from build123d import *

# Parameters (mm, degrees)
SKETCH_2_W          = 43.624420354
SKETCH_2_H          = 30
CUT_EXTRUDE_1_DEPTH = 9


with BuildPart() as part:
    # Эскиз1 → Повернуть1 (revolve)
    with BuildSketch(Plane(origin=(0, 0, 0), x_dir=(0, 0, -1), z_dir=(1, 0, 0))):
        Polygon((2.25, 26.387863371), (0, 26.387863371), (0, -1.191709959), (17.25, -1.191709959), (17.25, 65.340178843), (2.55, 65.340178843), (2.55, 50.340178843), (2.25, 50.340178843), align=None)
    revolve(axis=Axis((0, 93.464109616, 0), (0, -1, 0)))

    # Эскиз2 → Вырез-Вытянуть1 (cut)
    with BuildSketch(Plane.XY):
        with Locations((0, 65.340178843)):
            Rectangle(SKETCH_2_W, SKETCH_2_H)
    extrude(amount=-CUT_EXTRUDE_1_DEPTH, mode=Mode.SUBTRACT)


solid = part.part
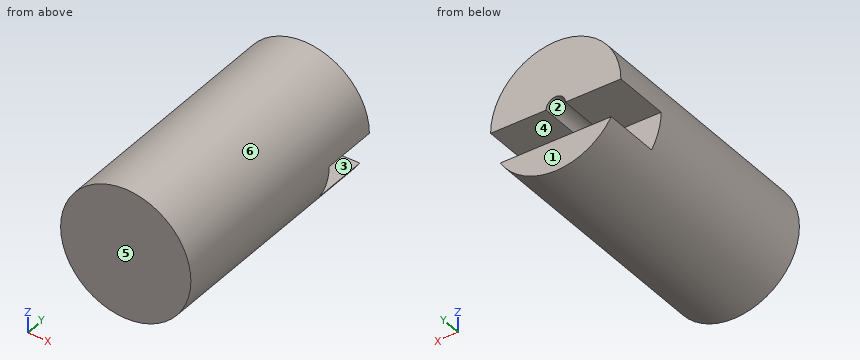
Can you work these out from the model? Positions are in its coordinate system, mm. Face numbers are marked on the shaded views. A direction names the side the tool comes from. Give positions to 0.01 mm unless a question says otherwise; leave off trailing zeros. Loops run counter-clockwise (first coordinate to the right, second up) from the corner with the lowest first, then second, coordinate; pieces in that order, holes last. Notation, with made-up numbers: (84.5, 11) -> (113.5, 11) arc R26 ccw to (113.5, 49) -> close; hole circle Ø3 at (30, -32.75). An arc over 180 degrees is marked (long way). Use one line per item in the form item = value.
1) Will these pins go through, and if not, where does the flat tip stop? pin 1 (1 mm diameter, centred on x = -9.5, y = 51, fed in from +Z); pin 2 (1.3 mm diameter, centred on x = 0, z = -0.5, fed in from +Y); pin 3 (7.5 mm diameter, centred on x = -9, y = 59, fed in from -Z).
Answers:
pin_1 = 14.72
pin_2 = 26.39
pin_3 = -16.43
2) I need wall thicknesses on line 1 along X through (y, z) = (42, 0); line 2 along Y through (x, z) = (6.5, -3). Which ranges of each line are inside material? Lowest first, please.
Answers:
line_1 = -17.25 to -2.25, 2.25 to 17.25
line_2 = -1.19 to 50.34
3) If we section it at D-D (x = 0): Please give me the cut outline in (y, z), plus the area to 3 significant figures.
Answers:
outline = (-1.19, -17.25) -> (65.34, -17.25) -> (65.34, -9) -> (50.34, -9) -> (50.34, -2.25) -> (26.39, -2.25) -> (26.39, 2.25) -> (50.34, 2.25) -> (50.34, 2.55) -> (65.34, 2.55) -> (65.34, 17.25) -> (-1.19, 17.25) -> close
area = 2,010 mm²
4) If we section it at B-B (x = -13.5): Please give me the cut outline in (y, z), plus the area to 3 significant figures.
Answers:
outline = (-1.19, -10.74) -> (65.34, -10.74) -> (65.34, -9) -> (50.34, -9) -> (50.34, 0) -> (65.34, 0) -> (65.34, 10.74) -> (-1.19, 10.74) -> close
area = 1,290 mm²
5) For the marked faces 1, 2 and 3, which set-ups out of +Z, -Z, +X, -X, +Y, -Y let a thin tool reach every point of the face, with its end or its side?
Answers:
face_1 = +Z, -Z, +X, -X, +Y
face_2 = +Y
face_3 = +X, -X, +Y
6) We'd pull the mould along Z, two halves only. Please class the marked faces 4, 5 and 6: released by +Z, released by -Z, zero draft, split by the parting line, or undercut.
Answers:
face_4 = undercut
face_5 = zero draft
face_6 = split by the parting line
7) If we section it at C-C (y = 8.5): Please give me the cut outline in (x, z), plus the area to 3 significant figures.
Answers:
outline = circle Ø34.5 at (0, 0)
area = 935 mm²
8) If we section it at A-A (y = 44.5): Please give me the cut outline in (x, z), plus the area to 3 significant figures.
Answers:
outline = circle Ø34.5 at (0, 0); hole circle Ø4.5 at (0, 0)
area = 919 mm²
